Study the drawing (mm; zero at the part's minimum x, y, z) and answer. Coordinates: 2 decimals unless noted, no trailing zeros. Order: outer loops, then holes, each group sorted by start corner. A loop starts at its lowest first (then second) coordinate and runs counter-clockwise, first axis right, second up.
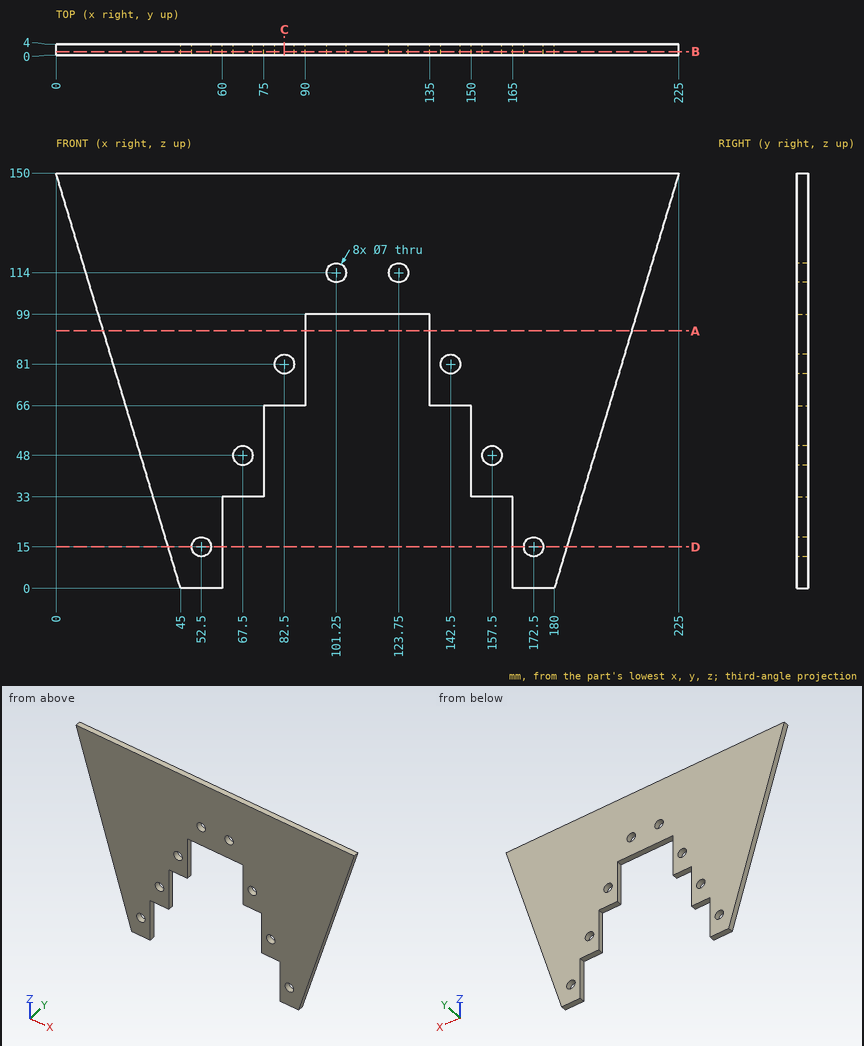
1) A cutting plane is placed at D-D, the plane z = 15. Determine the outline of the cut face in (x, y), and give its area (3 significant figures).
A:
outline: (40.5, 0) - (49, 0) - (49, 4) - (40.5, 4) - close; (56, 0) - (60, 0) - (60, 4) - (56, 4) - close; (165, 0) - (169, 0) - (169, 4) - (165, 4) - close; (176, 0) - (184.5, 0) - (184.5, 4) - (176, 4) - close
area: 100 mm2
2) Flat-ended cylindrical pins translate along their axes: pin 1 Ø2 at (y, z) = (2.5, 26.5) entering from +X; pin 2 Ø1.5 at (x, y) = (65, 1) entering from -Z. Find the tip coordinate at first contact, or state that the pin passes through.
A:
pin 1: stops at x = 188.25
pin 2: stops at z = 33
3) Straight lines are drawn through the part: line 1 (X direction, y = 1.55, z = 114); line 2 (X direction, y = 2.7, z = 81); line 3 (X direction, y = 2.5, z = 48). For each, find the intervals that lie inside material, in ascending order.
A:
line 1: x = 10.8 to 97.75, 104.75 to 120.25, 127.25 to 214.2
line 2: x = 20.7 to 79, 86 to 90, 135 to 139, 146 to 204.3
line 3: x = 30.6 to 64, 71 to 75, 150 to 154, 161 to 194.4
4) A cutting plane is placed at B-B, the plane y = 1.25. State how many separate pieces and enclosed holes the cut face has, and give its area (3 significant figures).
A:
separate pieces: 1
enclosed holes: 8
area: 19,300 mm2
5) A cutting plane is placed at A-A, the plane z = 93. Determine the outline of the cut face in (x, y).
A:
outline: (17.1, 0) - (90, 0) - (90, 4) - (17.1, 4) - close; (135, 0) - (207.9, 0) - (207.9, 4) - (135, 4) - close
6) A cutting plane is placed at C-C, the plane x = 82.5. Determine the outline of the cut face in (y, z), and give its area (3 significant figures).
A:
outline: (0, 66) - (4, 66) - (4, 77.5) - (0, 77.5) - close; (0, 84.5) - (4, 84.5) - (4, 150) - (0, 150) - close
area: 308 mm2
